Read the model definition and answer for the solid it produces. Units are mm, in the model's axes. A direction names the side the tool comes from. Round coordinates to 2 decimals unless told otherwise and drop trailing zeros. Order: outer loops, then holes, each group sorted by start corner. A loop starts at its lowest first (then second) coordinate and runs counter-clockwise, first axis right, second up. Notation, with made-up numbers: (51, 1.25) -> (82, 1.25) arc R24 ccw to (82, 19.25) -> close; hole circle Ø9 at (38, 3.5). An arc over 180 degrees is marked (long way). Answer as a JSON object with one key per item and string values. Group by question number.
Item 1: Given P1, Ø5, axis at x = -5.5, z = 5.5, coming from the -Y side; P2, Ø5, axis at x = 2, z = 1, coming from the +Y side; P3, Ø5, axis at x = -9, z = 6, coming from the +Y side; P4, Ø4, axis at x = 11, z = 1.5, coming from the +Y side, each flat-ended and moving along its own axis, determine where each tip first touches the part or whether it passes through.
Item 2: Section B-B, the plane x = 0 is taken. Write down the section's boundary in (y, z).
Item 3: Section C-C, the plane z = 8.25 is taken. Write down the section's boundary in (x, y).
Item 4: The mould has two halves that part along X. Classify faces 3 (the cylindrical face through (0, 57, 5)), 4 (the flat face through (14.5, 9, 5)), 5 (the flat face through (0, 0, 5)): pulls with the +X half, pulls with the -X half, needs draft (parallel to the pull), parting line crosses it, or undercut.
Item 5: For faces 1 (the flat face through (12.5, -11, 5)), 2 (the flat face through (-14.5, 10, 5)), determine the directions among +Z, -Z, +X, -X, +Y, -Y from which every point of the face is accessible in a straight line to the end or side of a thin tool.
Item 6: Section A-A, the plane y = -4 is taken. Write down the section's boundary in (x, z).
Item 7: Consider probe 1 along X at (y, z) = (-11, 2); probe 2 along Y at (x, z) = (0, 5.5); probe 3 along X at (y, z) = (46, 3.25). Determine where each line is inside the solid, lowest interval first. Write a range as from..to.
from build123d import *

# Parameters (mm, degrees)
F2_DEPTH = 10
F1_R     = 13.5
F3_DEPTH = 10


with BuildPart() as f2:
    # F0 (on Top) → F2 (new body)
    with BuildSketch(Plane.XY):
        Polygon((-12.5, 0), (12.5, 0), (14.5, 0), (14.5, 28), (0, 28), (-14.5, 28), (-14.5, 0), align=None)
        with BuildLine():
            Line((14.5, 0), (12.5, 0))
            Line((12.5, 0), (12.5, -21.5167603026))
            ThreePointArc((12.5, -21.5167603026), (13.8733092656, -21.7550100402), (14.5, -23))
            Line((14.5, -23), (14.5, 0))
        make_face()
        with BuildLine():
            ThreePointArc((14.5, -23), (13.8733092656, -21.7550100402), (12.5, -21.5167603026))
            Line((12.5, -21.5167603026), (12.5, -23))
            Line((12.5, -23), (14.5, -23))
        make_face()
        with BuildLine():
            Line((12.5, -23), (12.5, -21.5167603026))
            ThreePointArc((12.5, -21.5167603026), (12.0266907344, -24.2449899598), (14.5, -23))
            Line((14.5, -23), (12.5, -23))
        make_face()
        with BuildLine():
            Line((-12.5, -21.5167603026), (-12.5, 0))
            Line((-12.5, 0), (-14.5, 0))
            Line((-14.5, 0), (-14.5, -23))
            ThreePointArc((-14.5, -23), (-13.8733092656, -21.7550100402), (-12.5, -21.5167603026))
        make_face()
        with BuildLine():
            Line((0, 28), (14.5, 28))
            Line((14.5, 28), (14.5, 42.5))
            ThreePointArc((14.5, 42.5), (10.2530483272, 32.2469516728), (0, 28))
        make_face()
        with BuildLine():
            ThreePointArc((-11.4, -23), (-11.7050100402, -22.0766907344), (-12.5, -21.5167603026))
            Line((-12.5, -21.5167603026), (-12.5, -23))
            Line((-12.5, -23), (-14.5, -23))
            ThreePointArc((-14.5, -23), (-12.95, -24.55), (-11.4, -23))
        make_face()
        with BuildLine():
            Line((-12.5, -23), (-12.5, -21.5167603026))
            ThreePointArc((-12.5, -21.5167603026), (-13.8733092656, -21.7550100402), (-14.5, -23))
            Line((-14.5, -23), (-12.5, -23))
        make_face()
        with BuildLine():
            Line((-14.5, 28), (0, 28))
            ThreePointArc((0, 28), (-10.2530483272, 32.2469516728), (-14.5, 42.5))
            Line((-14.5, 42.5), (-14.5, 28))
        make_face()
        with BuildLine():
            ThreePointArc((-14.5, 42.5), (-10.2530483272, 32.2469516728), (0, 28))
            ThreePointArc((0, 28), (10.2530483272, 32.2469516728), (14.5, 42.5))
            ThreePointArc((14.5, 42.5), (0, 57), (-14.5, 42.5))
        make_face()
    extrude(amount=F2_DEPTH)

    # F1 (on Top) → F3 (cut)
    with BuildSketch(Plane.XY):
        with Locations((0, 41.5)):
            Circle(F1_R)
    extrude(amount=F3_DEPTH, mode=Mode.SUBTRACT)


solid = f2.part
Values found:
{
 "1": {"P1": "y = 0", "P2": "y = 57", "P3": "y = 55.46", "P4": "y = 53.87"},
 "2": {"outline": "(0, 0) -> (28, 0) -> (28, 10) -> (0, 10) -> close; (55, 0) -> (57, 0) -> (57, 10) -> (55, 10) -> close"},
 "3": {"outline": "(-14.5, -23) arc R1.55 ccw (long way) to (-12.5, -21.52) -> (-12.5, 0) -> (12.5, 0) -> (12.5, -21.52) arc R1.55 ccw (long way) to (14.5, -23) -> (14.5, 42.5) arc R14.5 ccw to (-14.5, 42.5) -> close; hole circle Ø27 at (0, 41.5)"},
 "4": {"face 3": "parting line crosses it", "face 4": "pulls with the +X half", "face 5": "undercut"},
 "5": {"face 1": "+Z, -Z", "face 2": "+Z, -Z, -X, +Y, -Y"},
 "6": {"outline": "(-14.5, 0) -> (-12.5, 0) -> (-12.5, 10) -> (-14.5, 10) -> close; (12.5, 0) -> (14.5, 0) -> (14.5, 10) -> (12.5, 10) -> close"},
 "7": {"probe 1": "-14.5..-12.5, 12.5..14.5", "probe 2": "0..28, 55..57", "probe 3": "-14.07..-12.73, 12.73..14.07"}
}
